```python
from build123d import *

# Parameters (mm, degrees)
F1_DEPTH = 8
F3_W     = 8
F3_H     = 8
F3_R     = 2.4
F4_DEPTH = 1.7
F5_R     = 2.4
F6_DEPTH = 1.7


with BuildPart() as f1:
    # F0 (on Front) → F1 (new body)
    with BuildSketch(Plane.XZ):
        Polygon((-2.4, 9.6), (-4, 9.6), (-4, 0), (4, 0), (4, 9.6), (2.4, 9.6), (2.4, 11.3), (-2.4, 11.3), align=None)
    extrude(amount=F1_DEPTH)

    # F3 (on plane+point) → F4 (cut, through all)
    with BuildSketch(Plane.XY.offset(11.3)):
        with Locations((0, -4)):
            Rectangle(F3_W, F3_H)
        with Locations((0, -4)):
            Circle(F3_R, mode=Mode.SUBTRACT)
    extrude(amount=-F4_DEPTH, mode=Mode.SUBTRACT)

    # F5 (on Top) → F6 (cut)
    with BuildSketch(Plane.XY):
        with Locations((0, -4)):
            Circle(F5_R)
    extrude(amount=F6_DEPTH, mode=Mode.SUBTRACT)


solid = f1.part
```
Here's how the part is built. I have some questions about the finished solid (model axes, mm). A direction names the side the tool comes from. Coordinates: 2 decimals unless noted, no trailing zeros. Write each loop counter-clockwise with the first axis right and the second up, starting at its lowest first coordinate (ties: lowest second). Pieces come first, ordered by that corner, then holes. Notation, with made-up numbers: M 2.25,16 L 17.25,16 A20 cw 17.25,32 Z; hole C 20,23.5 d9. An arc over 180 degrees is marked long. Answer as CSV lines item,"result". Start each with the question number.
Q1. Suppose I cut it at C-C, the plane z = 10.25. List the corners of the cut face in (x, y) for me, then the cut area to 3 significant figures.
Q2. Will this pin go through, and if not, where does the flat tip stop? pin 1 Ø1.4 at (x, y) = (0.5, -3.5) entering from -Z.
Q3. If we mould it in two halves opening along X, with no side actions, what happens to faces 1 (the cylindrical face through (1.29, -1.976, 0.838)), 2 (the flat face through (-4, -4, 5)), 3 (the flat face through (0, 0, 5))? For each: pulls with the +X half, pulls with the -X half, needs draft (parallel to the pull), parting line crosses it, or undercut.
Q4. Suppose I cut it at B-B, the plane y = -4. List the corners of the cut face in (x, z) for me.
Q5. Suppose I cut it at A-A, the plane x = 0. List the corners of the cut face in (y, z) for me, then the cut area to 3 significant figures.
Q6. For faces 4 (the flat face through (-2, -6, 9.6)), 5 (the flat face through (0, -4, 1.7)), 6 (the flat face through (0, -4, 11.3)), which set-ups out of +Z, -Z, +X, -X, +Y, -Y let a thin tool reach every point of the face, with its end or its side?
Q7. I need wall thicknesses on probe 1 along Y at (x, z) = (0, 0.7); probe 2 along Z at (x, y) = (-3, -3.5); probe 3 along Z at (x, y) = (2, -3). Which ranges of each line are inside material? Lowest first, please. Write a range as [from, to].
Entries:
1,outline,"C 0,-4 d4.8"
1,area,"18.1 mm²"
2,pin 1,"stops at z = 1.7"
3,face 1,"undercut"
3,face 2,"pulls with the -X half"
3,face 3,"needs draft"
4,outline,"M -4,0 L -2.4,0 L -2.4,1.7 L 2.4,1.7 L 2.4,0 L 4,0 L 4,9.6 L 2.4,9.6 L 2.4,11.3 L -2.4,11.3 L -2.4,9.6 L -4,9.6 Z"
5,outline,"M -8,0 L -6.4,0 L -6.4,1.7 L -1.6,1.7 L -1.6,0 L 0,0 L 0,9.6 L -1.6,9.6 L -1.6,11.3 L -6.4,11.3 L -6.4,9.6 L -8,9.6 Z"
5,area,"76.8 mm²"
6,face 4,"+Z"
6,face 5,"-Z"
6,face 6,"+Z, +X, -X, +Y, -Y"
7,probe 1,"y = [-8, -6.4], [-1.6, 0]"
7,probe 2,"z = [0, 9.6]"
7,probe 3,"z = [1.7, 11.3]"
